Autodesk Inventor part; units mm, degrees
ref_plane "YZ Plane" through (0, 0, 0) normal (1, 0, 0) x (0, 1, 0)
ref_plane "XZ Plane" through (0, 0, 0) normal (0, 1, 0) x (-1, 0, 0)
ref_plane "XY Plane" through (0, 0, 0) normal (0, 0, 1) x (1, 0, 0)
sketch "Sketch1" plane through (0, 0, 0) normal (0, 0, 1) x (1, 0, 0)
  line L0 (22.7021, 34.3404) -> (19.7021, 34.3404)
  line L1 (19.7021, 34.3404) -> (19.7021, 28.7404)
  line L2 (19.7021, 28.7404) -> (9.3021, 5.3404)
  line L3 (22.7021, 28.1038) -> (11.2517, 2.3404)
  line L4 (9.3021, 5.3404) -> (3.7021, 5.3404)
  line L5 (3.7021, 5.3404) -> (3.7021, 2.3404)
  line L6 (22.7021, 34.3404) -> (22.7021, 28.1038)
  line L7 (3.7021, 2.3404) -> (11.2517, 2.3404)
  point P0 (0, 0)
  dimension "d0" = 3
  dimension "d1" = 3
  dimension "d2" = 32
  dimension "d3" = 19
  dimension "d4" = 5.6
  dimension "d5" = 5.6
  dimension "d6" = 3
extrude "Extrusion1" add sketch "Sketch1" along normal blind 42
sketch "Sketch2" plane through (3.7021, 5.3404, 0) normal (0, 1, 0) x (1, 0, 0)
  line L0 (0, -42) -> (5.6, -42)
  circle A0 centre (2.8, -4) radius 1.35
  circle A1 centre (2.8, -21) radius 1.35
  circle A2 centre (2.8, -38) radius 1.35
  point P0 (-3.7021, 0)
  dimension "d9" = 2.7
  dimension "d10" = 2.7
  dimension "d11" = 2.7
  dimension "d12" = 17
  dimension "d13" = 17
  dimension "d14" = 4
extrude "Extrusion2" cut sketch "Sketch2" against normal through all
sketch "Sketch3" plane through (19.7021, 28.7404, 0) normal (-1, 0, 0) x (0, 0, 1)
  line L0 (0, 5.6) -> (42, 5.6)
  line L1 (0, 5.6) -> (0, 0)
  circle A0 centre (4, 2.8) radius 1.35
  circle A1 centre (21, 2.8) radius 1.35
  circle A2 centre (38, 2.8) radius 1.35
  point P0 (0, -28.7404)
  dimension "d17" = 2.7
  dimension "d18" = 2.7
  dimension "d19" = 2.7
  dimension "d20" = 17
  dimension "d21" = 17
  dimension "d22" = 4
  dimension "d23" = 2.8
  dimension "d24" = 2.8
  dimension "d25" = 2.8
extrude "Extrusion3" cut sketch "Sketch3" against normal through all
properties part number "Trunk" material "Aluminum-6061"
Work out the finished part from the listing and answer in its coordinate system (mm). A direction names the side the tool comes from. Coordinates: 2 decimals unless noted, no trailing zeros. Write each loop counter-clockwise with the first axis right and the second up, starting at its lowest first coordinate (ties: lowest second). Pieces come first, ordered by that corner, then holes. Notation, with made-up numbers: M -26.5,10 L 6.5,10 A10 cw 6.5,20 Z; hole C 0,41.25 d1. An arc over 180 degrees is marked long. Use one line per item in the form item = value. Start each with the question number.
1. A tool of negligible diameter and unlimited length cuts with its end or side. For faces 1 (the face through (7.125, 3.861, 22.198)), 2 (the face through (19.702, 30, 21)), from which of +Z, -Z, +X, -X, +Y, -Y can it reach the whole face along a straight path? Write none if from no direction.
2. The part is cut by section A-A (z = 4). Give the vertices of the cut face in (x, y).
3. The part is cut by section D-D (x = 21.25). Give the vertices of the cut face in (y, z), plus the area to 3 significant figures.
4. The part is cut by section B-B (x = 7). Give the vertices of the cut face in (y, z).
5. The part is cut by section C-C (z = 10.5). Give the vertices of the cut face in (x, y).
6. The mould has two halves that part along Y. Classify faces 3 (the face through (21.181, 32.679, 38.726)), 4 (the face through (21.18, 32.88, 3.82)), 5 (the face through (3.702, 4, 21)), 6 (the face through (14.575, 17.204, 20.706)): released by +Y, released by -Y, zero draft, split by the parting line, or undercut.
7. Each of these flat-tipped pins is pushed along its axis until it touches: P1, Ø3, axis at y = 32, z = 22.5, coming from the -X side; P2, Ø12, axis at y = 12.5, z = 21, coming from the -X side; P3, Ø1, axis at y = 7.5, z = 10.5, coming from the +X side. Where does it stop, or does it pass through?
8. Straight lines are drawn through the part: probe 1 along X at (y, z) = (30.5, 2); probe 2 along Y at (x, z) = (6.5, 28); probe 3 along Y at (x, z) = (19.75, 4.5). For each, find the intervals that lie inside material, in ascending order. Write a range as from..to.
Evaluation:
q1.face_1 = +Y, -Y
q1.face_2 = +Z, -Z, -X, +Y
q2.outline = M 3.7,2.34 L 5.15,2.34 L 5.15,5.34 L 3.7,5.34 Z; M 7.85,2.34 L 11.25,2.34 L 22.7,28.1 L 22.7,30.19 L 19.7,30.19 L 19.7,28.74 L 9.3,5.34 L 7.85,5.34 Z; M 19.7,32.89 L 22.7,32.89 L 22.7,34.34 L 19.7,34.34 Z
q3.outline = M 24.84,0 L 34.34,0 L 34.34,42 L 24.84,42 Z; hole C 31.54,4 d2.7; hole C 31.54,21 d2.7; hole C 31.54,38 d2.7
q3.area = 382 mm^2
q4.outline = M 2.34,0 L 5.34,0 L 5.34,2.75 L 2.34,2.75 Z; M 2.34,5.25 L 5.34,5.25 L 5.34,19.75 L 2.34,19.75 Z; M 2.34,22.25 L 5.34,22.25 L 5.34,36.75 L 2.34,36.75 Z; M 2.34,39.25 L 5.34,39.25 L 5.34,42 L 2.34,42 Z
q5.outline = M 3.7,2.34 L 11.25,2.34 L 22.7,28.1 L 22.7,34.34 L 19.7,34.34 L 19.7,28.74 L 9.3,5.34 L 3.7,5.34 Z
q6.face_3 = undercut
q6.face_4 = undercut
q6.face_5 = zero draft
q6.face_6 = released by +Y
q7.P1 = 19.7
q7.P2 = 9.82
q7.P3 = 13.77
q8.probe_1 = 19.7..22.7
q8.probe_2 = 2.34..5.34
q8.probe_3 = 21.46..30.29, 32.79..34.34
